Here's how the part is built. I have some questions about the finished solid (model axes, mm). A direction names the side the tool comes from. Round coordinates to 2 decimals unless told otherwise and drop trailing zeros. Write each loop counter-clockwise with the first axis right and the second up, starting at its lowest first coordinate (ties: lowest second). Pieces come first, ordered by that corner, then holes. Notation, with made-up numbers: (86, 49.5) -> (145, 49.5) arc R21 cw to (145, 55.5) -> close; hole circle Ø8 at (11, 19.25). An arc over 180 degrees is marked (long way). Put each result on its own line as item: value. Start each with the question number.
1. I need wall thicknesses on probe 1 along Z at (x, y) = (-27.8, -20); probe 2 along Z at (x, y) = (-20, -28); probe 3 along Y at (x, z) = (4, 132). Which ranges of each line are inside material? Lowest first, please. Write a range as from..to.
2. Suppose I cut it at A-A (y = -20). Please give me the cut outline in (x, z), then the cut area to 3 significant figures.
3. For pin 1 (5 mm diameter, centred on y = -20, z = 190, fed in from -X); pin 2 (6.5 mm diameter, centred on y = 20, z = 150, fed in from -X), each with a flat end and sliding along its axis, tell me the tip position at first contact or that it passes through.
4. Suppose I cut it at C-C (y = 7.5). Please give me the cut outline in (x, z), then the cut area to 3 significant figures.
5. Which directions (+Z, -Z, +X, -X, +Y, -Y) give clear straight access to the entire face, cutting with the end or side of a thin tool? Please do faces 4 (the face through (27, 0, 99)), 5 (the face through (-20.358, -28.521, 52.727)), 6 (the face through (-2, -29, 200)), 7 (the face through (-28.521, 20.358, 72.727)).
6. Suppose I cut it at B-B (x = -20). Please give me the cut outline in (y, z), then the cut area to 3 significant figures.
7. Suppose I cut it at D-D (z = 24.5). Please give me the cut outline in (x, y), then the cut area to 3 significant figures.
8. We'd pull the mould along X, two halves only. Please class faces 1 (the face through (-30, 0, 99)), 2 (the face through (17.253, -28.521, 10.121)), 3 (the face through (-28.521, 20.596, 107.315)): +X half, -X half, draft (parallel to the pull), parting line (faces both ways), or undercut.
```python
from build123d import *

# Parameters (mm, degrees)
SKETCH_W        = 60
SKETCH_H        = 60
SKETCH_W_2      = 54
SKETCH_H_2      = 54
PAD_DEPTH       = 200
SKETCH001_R     = 2.75
POCKET_DEPTH    = 3
SKETCH002_R     = 2.75
POCKET001_DEPTH = 3


with BuildPart() as part:
    # Sketch → Pad (new body)
    with BuildSketch(Plane.XY):
        Rectangle(SKETCH_W, SKETCH_H)
        Rectangle(SKETCH_W_2, SKETCH_H_2, mode=Mode.SUBTRACT)
    extrude(amount=PAD_DEPTH)

    # Sketch001 (on Face3 of Pad) → Pocket (cut)
    with BuildSketch(Plane.XZ.offset(30)):
        with Locations((-20, 50)):
            Circle(SKETCH001_R)
        with Locations((20, 50)):
            Circle(SKETCH001_R)
        with Locations((-20, 10)):
            Circle(SKETCH001_R)
        with Locations((20, 10)):
            Circle(SKETCH001_R)
    extrude(amount=-POCKET_DEPTH, mode=Mode.SUBTRACT)

    # Sketch002 (on Face2 of Pocket) → Pocket001 (cut)
    with BuildSketch(Plane(origin=(-30, 0, 0), x_dir=(0, -1, 0), z_dir=(-1, 0, 0))):
        with Locations((-20, 190)):
            Circle(SKETCH002_R)
        with Locations((20, 190)):
            Circle(SKETCH002_R)
        with Locations((-20, 150)):
            Circle(SKETCH002_R)
        with Locations((-60, 150)):
            Circle(SKETCH002_R)
        with Locations((-20, 110)):
            Circle(SKETCH002_R)
        with Locations((20, 110)):
            Circle(SKETCH002_R)
        with Locations((-20, 70)):
            Circle(SKETCH002_R)
        with Locations((20, 70)):
            Circle(SKETCH002_R)
    extrude(amount=-POCKET001_DEPTH, mode=Mode.SUBTRACT)


solid = part.part
```
Verdict:
1. probe 1: z = 0..67.25, 72.75..107.25, 112.75..187.25, 192.75..200
1. probe 2: z = 0..7.25, 12.75..47.25, 52.75..200
1. probe 3: y = -30..-27, 27..30
2. outline: (-30, 0) -> (-27, 0) -> (-27, 67.25) -> (-30, 67.25) -> close; (-30, 72.75) -> (-27, 72.75) -> (-27, 107.25) -> (-30, 107.25) -> close; (-30, 112.75) -> (-27, 112.75) -> (-27, 187.25) -> (-30, 187.25) -> close; (-30, 192.75) -> (-27, 192.75) -> (-27, 200) -> (-30, 200) -> close; (27, 0) -> (30, 0) -> (30, 200) -> (27, 200) -> close
2. area: 1,150 mm^2
3. pin 1: stops at x = 27
3. pin 2: stops at x = -30
4. outline: (-30, 0) -> (-27, 0) -> (-27, 200) -> (-30, 200) -> close; (27, 0) -> (30, 0) -> (30, 200) -> (27, 200) -> close
4. area: 1,200 mm^2
5. face 4: +Z, -Z
5. face 5: -Y
5. face 6: +Z, +X, -X, +Y, -Y
5. face 7: -X
6. outline: (-30, 0) -> (-27, 0) -> (-27, 7.25) -> (-30, 7.25) -> close; (-30, 12.75) -> (-27, 12.75) -> (-27, 47.25) -> (-30, 47.25) -> close; (-30, 52.75) -> (-27, 52.75) -> (-27, 200) -> (-30, 200) -> close; (27, 0) -> (30, 0) -> (30, 200) -> (27, 200) -> close
6. area: 1,170 mm^2
7. outline: (-30, -30) -> (30, -30) -> (30, 30) -> (-30, 30) -> close; hole (-27, -27) -> (27, -27) -> (27, 27) -> (-27, 27) -> close
7. area: 684 mm^2
8. face 1: -X half
8. face 2: undercut
8. face 3: draft
